For this review, take the finished solid that the model builds, in its own axes (mm). Face numbers are marked on the shaded views. A direction names the side the tool comes from. Give positions to 0.01 mm unless a question says otherwise; leave off trailing zeros. Loops run counter-clockwise (first coordinate to the right, second up) from the corner with the lowest first, then second, coordinate; pieces in that order, holes last. Notation, with made-up numbers: (28, -31) - (41, -31) arc R19 ccw to (41, -7) - close; hole circle Ø1 at (8, 73). An arc over 180 degrees is marked (long way). Answer in a Markdown table with one row per item.
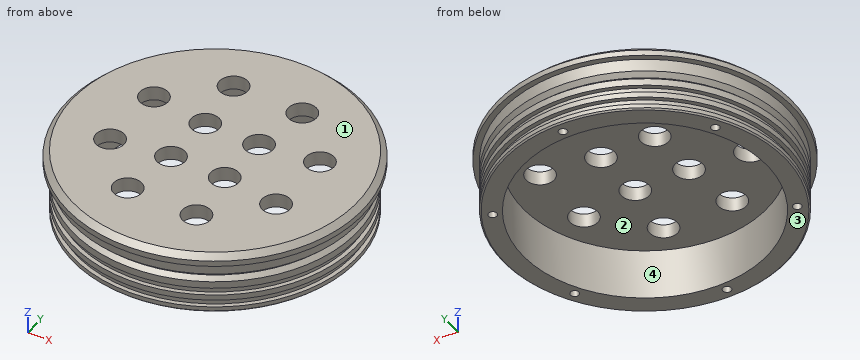
```python
from build123d import *

# Parameters (mm, degrees)
CHAMFER_1_SIZE      = 2
SKETCH_4_R          = 5
CUT_EXTRUDE_2_DEPTH = 10
SKETCH_5_R          = 1.5
CUT_EXTRUDE_3_DEPTH = 10


with BuildPart() as part:
    # Эскиз2 → Повернуть1 (revolve)
    with BuildSketch(Plane(origin=(0, 0, 0), x_dir=(1, 0, 0), z_dir=(0, 1, 0)), mode=Mode.PRIVATE) as revolve_1_sk:
        Polygon((0, 0), (0, 5), (-43.5, 5), (-43.5, 23.2), (-50, 23.2), (-50.5, 22.7), (-50.5, 21.2), (-49, 21.2), (-49, 18.6), (-50.5, 18.6), (-50.5, 16.6), (-49, 16.6), (-49, 14), (-50.5, 14), (-50.5, 11.5), (-49, 10), (-50.5, 8.5), (-50.5, 4), (-52.5, 4), (-52.5, 0), (-18.386389901, 0), align=None)
    revolve(revolve_1_sk.sketch.rotate(Axis((0, 0, 0), (0, 0, -1)), 180), axis=Axis((0, 0, 0), (0, 0, -1)))

    # Фаска1
    chamfer_1_edges = [part.edges().sort_by_distance(p)[0] for p in [
        (-52.5, 0, 0),
    ]]
    chamfer(chamfer_1_edges, length=CHAMFER_1_SIZE)

    # Эскиз4 → Вырез-Вытянуть2 (cut)
    with BuildSketch(Plane.XY):
        with Locations((-12.437211552, -30.026084807)):
            Circle(SKETCH_4_R)
        with Locations((-30.026084807, 12.437211552)):
            Circle(SKETCH_4_R)
        with Locations((-12.437211552, 30.026084807)):
            Circle(SKETCH_4_R)
        with Locations((12.437211552, 30.026084807)):
            Circle(SKETCH_4_R)
        with Locations((30.026084807, 12.437211552)):
            Circle(SKETCH_4_R)
        with Locations((30.026084807, -12.437211552)):
            Circle(SKETCH_4_R)
        with Locations((12.437211552, -30.026084807)):
            Circle(SKETCH_4_R)
        with Locations((-30.026084807, -12.437211552)):
            Circle(SKETCH_4_R)
        with Locations((-9.722718241, 9.722718241)):
            Circle(SKETCH_4_R)
        with Locations((9.722718241, 9.722718241)):
            Circle(SKETCH_4_R)
        with Locations((9.722718241, -9.722718241)):
            Circle(SKETCH_4_R)
        with Locations((-9.722718241, -9.722718241)):
            Circle(SKETCH_4_R)
    extrude(amount=-CUT_EXTRUDE_2_DEPTH, mode=Mode.SUBTRACT)

    # Эскиз5 → Вырез-Вытянуть3 (cut)
    with BuildSketch(Plane(origin=(0, 0, -23.2), x_dir=(-1, 0, 0), z_dir=(0, 0, -1))):
        with Locations((0, 46.5)):
            Circle(SKETCH_5_R)
        with Locations((40.270181276, 23.25)):
            Circle(SKETCH_5_R)
        with Locations((40.270181276, -23.25)):
            Circle(SKETCH_5_R)
        with Locations((0, -46.5)):
            Circle(SKETCH_5_R)
        with Locations((-40.270181276, -23.25)):
            Circle(SKETCH_5_R)
        with Locations((-40.270181276, 23.25)):
            Circle(SKETCH_5_R)
    extrude(amount=-CUT_EXTRUDE_3_DEPTH, mode=Mode.SUBTRACT)


solid = part.part
```
1. Wall thickness on line 1 (Y direction, x = 0, z = -19.5); line 2 (Z direction, x = -44.5, y = -23.5); line 3 (Z direction, x = -25, y = 4): over which ranges is each line inside the solid? List them lowest first. Write a range as [from, to].
Values:
| item | result |
|---|---|
| line 1 | y = [-49, -48], [-45, -43.5], [43.5, 45], [48, 49] |
| line 2 | z = [-22.88, -21.2], [-18.6, -16.6], [-14, -11.32], [-8.68, 0] |
| line 3 | z = [-5, 0] |
2. Mouldability with a two-part tool opening along Y and no side actions: class the marked faces 1 and 2 as released by +Y, released by -Y, zero draft, split by the parting line, or undercut.
Values:
| item | result |
|---|---|
| face 1 | zero draft |
| face 2 | undercut |
3. For the marked faces 3 and 4, list the 3-axis set-ups (+Z, -Z, +X, -X, +Y, -Y) from which the entire face can be reached by the end or side of a thin tool; tool diameter is ignored.
Values:
| item | result |
|---|---|
| face 3 | -Z, +X, -X, +Y, -Y |
| face 4 | -Z |
4. Clearance check with flat-ended pins moving along their axes: pin 1 (2.5 mm diameter, centred on x = 0, y = 46.5, fed in from -Z); pin 2 (9 mm diameter, centred on x = -30.03, y = -12.44, fed in from +Z); pin 3 (4 mm diameter, centred on x = 13, y = 9.5, fed in from -Z); pin 4 (12 mm diameter, centred on x = 2.5, z = -20.5, fed in from +Y). State where each tip first meets the part, or that it passes through.
Values:
| item | result |
|---|---|
| pin 1 | stops at z = -13.2 |
| pin 2 | passes through |
| pin 3 | stops at z = -5 |
| pin 4 | stops at y = 50.5 |
5. We need section A-A, the plane z = -6.5. Give the boundary of the cut face in (x, y), and give its area (3 significant figures).
Values:
| item | result |
|---|---|
| outline | circle Ø101 at (0, 0); hole circle Ø87 at (0, 0) |
| area | 2,070 mm^2 |
6. We need section B-B, the plane x = 31. Count the separate pieces of the cut face and the enclosed holes in it, and give its area (3 significant figures).
Values:
| item | result |
|---|---|
| separate pieces | 3 |
| enclosed holes | 0 |
| area | 630 mm^2 |
